from build123d import *

# Parameters (mm, degrees)
SKETCH1_R           = 12.5
SKETCH1_R_2         = 11.5
BOSS_EXTRUDE1_DEPTH = 175
SKETCH2_R           = 1.55
CUT_EXTRUDE1_DEPTH  = 12.5
SKETCH3_R           = 1.55
CUT_EXTRUDE2_DEPTH  = 12.5


with BuildPart() as part:
    # Sketch1 → Boss-Extrude1 (new, symmetric)
    with BuildSketch(Plane.XY):
        Circle(SKETCH1_R)
        Circle(SKETCH1_R_2, mode=Mode.SUBTRACT)
    extrude(amount=BOSS_EXTRUDE1_DEPTH, both=True)

    # Sketch2 → Cut-Extrude1 (cut, symmetric)
    with BuildSketch(Plane(origin=(0, 0, 0), x_dir=(1, 0, 0), z_dir=(0, 1, 0))):
        with Locations(Location((0, 155, 0), (0, 0, 270))):
            Circle(SKETCH2_R)
    extrude(amount=CUT_EXTRUDE1_DEPTH, both=True, mode=Mode.SUBTRACT)

    # Sketch3 → Cut-Extrude2 (cut, symmetric)
    with BuildSketch(Plane(origin=(0, 0, 0), x_dir=(1, 0, 0), z_dir=(0, 1, 0))):
        with Locations(Location((0, -165, 0), (0, 0, 270))):
            Circle(SKETCH3_R)
    extrude(amount=CUT_EXTRUDE2_DEPTH, both=True, mode=Mode.SUBTRACT)


solid = part.part
Geometry check sheet. Reference: the model listing, model coordinates, mm. Give positions to 0.01 mm unless a question says otherwise; leave off trailing zeros. Order: outer loops, then holes, each group sorted by start corner. A loop starts at its lowest first (then second) coordinate and runs counter-clockwise, first axis right, second up. Notation, with made-up numbers: M -20,39.25 L 16,39.25 A9 ccw 16,51.25 Z; hole C -16,77.5 d11. An arc over 180 degrees is marked long. Use a Markdown table: item, result.
Item 1: Section check B-B (x = 7.75). Record the cut outline in (y, z), and give its area (3 significant figures).
Answers follow:
| item | result |
|---|---|
| outline | M -9.81,-175 L -8.5,-175 L -8.5,175 L -9.81,175 Z; M 8.5,-175 L 9.81,-175 L 9.81,175 L 8.5,175 Z |
| area | 918 mm2 |
Item 2: Section check C-C (z = -94.5). Record the cut outline in (x, y).
Answers follow:
| item | result |
|---|---|
| outline | C 0,0 d25; hole C 0,0 d23 |
Item 3: Section check A-A (y = 0). Record the cut outline in (x, z).
Answers follow:
| item | result |
|---|---|
| outline | M -12.5,-175 L -11.5,-175 L -11.5,175 L -12.5,175 Z; M 11.5,-175 L 12.5,-175 L 12.5,175 L 11.5,175 Z |
Item 4: Depth check by flat-ended pin: P1, Ø2, axis at y = 7.5, z = -66, coming from the -X side; P2, Ø2.5, axis at x = 0, z = 165, coming from the -Y side; P3, Ø6, axis at x = -4, z = 127.5, coming from the -Y side; P4, Ø2, axis at x = 9.5, z = -30, coming from the +Y side. Enter the tip coordinate at first touch or a pass-through.
Answers follow:
| item | result |
|---|---|
| P1 | stops at x = -10.68 |
| P2 | passes through |
| P3 | stops at y = -12.46 |
| P4 | stops at y = 9.17 |
Item 5: Draft check along Y on faces 1 (the cylindrical face through (-1.5, 11.4, -2.4)), 2 (the cylindrical face through (11.923, 3.755, 2.45)), 3 (the flat face through (11, -4, -175)). Enter one of: +Y half, -Y half, draft (parallel to the pull), parting line (faces both ways), or undercut.
Answers follow:
| item | result |
|---|---|
| face 1 | undercut |
| face 2 | parting line |
| face 3 | draft |
Item 6: Material ranges on line 1 along Z through (x, y) = (0, 12.15); line 2 along Y through (x, z) = (0, 31); line 3 along Y through (x, z) = (-1.5, 77), recorded low to high.
Answers follow:
| item | result |
|---|---|
| line 1 | z = -175 to -156.55, -153.45 to 163.45, 166.55 to 175 |
| line 2 | y = -12.5 to -11.5, 11.5 to 12.5 |
| line 3 | y = -12.41 to -11.4, 11.4 to 12.41 |
